Check sheet for the modelled part. Datum: model origin and axes. Units: mm. Give positions to 0.01 mm unless a question says otherwise; leave off trailing zeros. Order: outer loops, then holes, each group sorted by start corner. A loop starts at its lowest first (then second) coordinate and runs counter-clockwise, first axis right, second up. Notation, with made-up numbers: (29, 55) - (52, 55) arc R9 cw to (52, 70) - close; hole circle Ø9 at (-9, 67.5). An arc over 180 degrees is marked (long way). Answer in a Markdown table with one row per item.
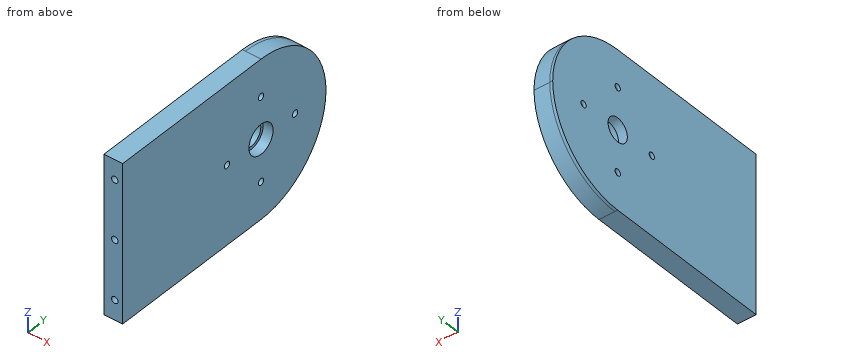
from build123d import *

# Parameters (mm, degrees)
STOCK_NEW_TRACKER_1_START = -68
STOCK_NEW_TRACKER_1_DEPTH = 8
SKETCH1_R                 = 7.5089999999999995
CUT_EXTRUDE1_DEPTH        = 5
SKETCH2_R                 = 6.000000000000002
CUT_EXTRUDE2_DEPTH        = 143.41825129942816
M4X0_7_TAPPED_HOLE1_D     = 3.3
M4X0_7_TAPPED_HOLE1_DEPTH = 35
M4X0_7_TAPPED_HOLE1_TIP   = 0.9914200213954745
M4X0_7_TAPPED_HOLE2_D     = 3.3
SKETCH10_R                = 1.6499999999999984
SKETCH10_R_2              = 1.6499999999999986
SKETCH10_R_3              = 6.000000000000005
BOSS_EXTRUDE1_DEPTH       = 1.5


# Read off the part's stored shape, not the designer's step: Stock-New_Tracker-1
with BuildPart() as part:
    # Stock-New_Tracker-1 outline → Stock-New_Tracker-1 (new body)
    with BuildSketch(Plane.YZ.offset(STOCK_NEW_TRACKER_1_START)):
        with BuildLine():
            Line((10, 40.00000001), (10, -40.00000001))
            Line((10, -40.00000001), (96.116983094, -40.00000001))
            ThreePointArc((96.116983094, -40.00000001), (124.570453888, -28.312888017), (136.594137145, 0))
            ThreePointArc((136.594137145, 0), (124.570453888, 28.312888017), (96.116983094, 40.00000001))
            Line((96.116983094, 40.00000001), (10, 40.00000001))
        make_face()
    extrude(amount=STOCK_NEW_TRACKER_1_DEPTH)

    # Sketch1 → Cut-Extrude1 (cut)
    with BuildSketch(Plane(origin=(-60, 0, 1.041e-14), x_dir=(-1.7e-16, 0, -1), z_dir=(1, 0, -1.7e-16))):
        with Locations((0, 96.11698309434121)):
            Circle(SKETCH1_R)
    extrude(amount=-CUT_EXTRUDE1_DEPTH, mode=Mode.SUBTRACT)

    # Sketch2 → Cut-Extrude2 (cut, through all)
    with BuildSketch(Plane(origin=(-65, 0, 1.128e-14), x_dir=(-1.7e-16, 0, -1), z_dir=(1, 0, -1.7e-16))):
        with Locations((0, 96.11698309434121)):
            Circle(SKETCH2_R)
    extrude(amount=-CUT_EXTRUDE2_DEPTH, mode=Mode.SUBTRACT)

    # M4x0.7 Tapped Hole1
    with Locations(Plane(origin=(0, 10, 0), x_dir=(-1, 0, 0), z_dir=(0, -1, 0))):
        with Locations((64, -30), (64, 0), (64, 30)):
            Hole(M4X0_7_TAPPED_HOLE1_D / 2, depth=M4X0_7_TAPPED_HOLE1_DEPTH)
            with Locations((0, 0, -(M4X0_7_TAPPED_HOLE1_DEPTH + M4X0_7_TAPPED_HOLE1_TIP / 2))):  # 118° drill point
                Cone(0, M4X0_7_TAPPED_HOLE1_D / 2, M4X0_7_TAPPED_HOLE1_TIP, mode=Mode.SUBTRACT)

    # M4x0.7 Tapped Hole2 (through all)
    with Locations(Plane.ZY.offset(67.99999999999999)):
        with Locations((0, 74.903779659), (-21.213203436, 96.116983094), (0, 117.33018653), (21.213203436, 96.116983094)):
            Hole(M4X0_7_TAPPED_HOLE2_D / 2)

    # Sketch10 → Boss-Extrude1 (add)
    with BuildSketch(Plane.ZY.offset(67.99999999999999)):
        with BuildLine():
            Line((40.00000000999996, 10), (40.00000000999996, 96.11698309434121))
            ThreePointArc((40.00000000999996, 96.11698309434121), (28.312888017242308, 124.57045388794387), (-3.291e-14, 136.59413714461505))
            ThreePointArc((-3.291e-14, 136.59413714461505), (-28.31288801724237, 124.57045388794387), (-40.00000001000003, 96.11698309434121))
            Line((-40.00000001000003, 96.11698309434121), (-40.00000001000003, 10))
            Line((-40.00000001000003, 10), (40.00000000999996, 10))
        make_face()
        with Locations((1.335e-14, 117.33018652993762)):
            Circle(SKETCH10_R, mode=Mode.SUBTRACT)
        with Locations((21.213203435596416, 96.11698309434121)):
            Circle(SKETCH10_R_2, mode=Mode.SUBTRACT)
        with Locations(Location((0, 96.11698309434121, 0), (0, 0, 180))):
            Circle(SKETCH10_R_3, mode=Mode.SUBTRACT)
        with Locations((-21.213203435596416, 96.11698309434121)):
            Circle(SKETCH10_R_2, mode=Mode.SUBTRACT)
        with Locations((1.513e-14, 74.9037796587448)):
            Circle(SKETCH10_R, mode=Mode.SUBTRACT)
    extrude(amount=BOSS_EXTRUDE1_DEPTH)


solid = part.part
(1) Cross-section at A-A, the plane y = 27.5. Record the cut outline in (x, z).
Geometry says:
| item | result |
|---|---|
| outline | (-69.5, -40) - (-60, -40) - (-60, 40) - (-69.5, 40) - close; hole circle Ø3.3 at (-64, -30); hole circle Ø3.3 at (-64, 0); hole circle Ø3.3 at (-64, 30) |
(2) Gauge pin test, flat ends, axial feed: P1, Ø4.5, axis at y = 96.12, z = 21.21, coming from the -X side; P2, Ø9.5, axis at y = 96.12, z = 0, coming from the +X side; P3, Ø13.5, axis at y = 96.12, z = 0, coming from the +X side; P4, Ø5, axis at x = -68.5, z = 19, coming from the +Y side. Record the tip position at first contact, or that the pin passes through.
Geometry says:
| item | result |
|---|---|
| P1 | x = -69.5 |
| P2 | through |
| P3 | x = -65 |
| P4 | y = 132.86 |
(3) Cross-section at C-C, the plane z = -14. Record the cut outline in (x, y), then the cut area to 3 significant figures.
Geometry says:
| item | result |
|---|---|
| outline | (-69.5, 10) - (-60, 10) - (-60, 133.92) - (-69.5, 133.92) - close |
| area | 1,180 mm² |
(4) Cross-section at B-B, the plane z = 33.5. Record the cut outline in (x, y), then the cut area to 3 significant figures.
Geometry says:
| item | result |
|---|---|
| outline | (-69.5, 10) - (-60, 10) - (-60, 118.12) - (-69.5, 118.12) - close |
| area | 1,030 mm² |
(5) Thickness scan on L1, parallel to X at y = 28, z = 30; L2, parallel to Y at x = -68.75, z = 20.5; L3, parallel to Y at x = -66, z = -21. Record the ranges inside material, lowest first.
Geometry says:
| item | result |
|---|---|
| L1 | -69.5 to -65.65, -62.35 to -60 |
| L2 | 10 to 94.63, 97.6 to 130.74 |
| L3 | 10 to 94.48, 97.75 to 130.43 |
